Build history of the part. All positions in model axes, mm. A direction names the side the tool comes from. Round coordinates to 2 decimals unless told otherwise and drop trailing zeros. Order: outer loops, then holes, each group sorted by start corner. A loop starts at its lowest first (then second) coordinate and runs counter-clockwise, first axis right, second up. Notation, with made-up numbers: (27.5, 6) -> (78.5, 6) arc R24 ccw to (78.5, 25) -> close; hole circle Ø10 at (76.5, 80). An arc over 180 degrees is marked (long way). Answer as a JSON object with one key per item and string values.
from build123d import *

# Parameters (mm, degrees)
F1_DEPTH = 12.7
F3_D     = 12.7


# Not quite as in the source:
# - a length typed as a fraction of an inch, garbled in the dataset ("3 / 203.2 mm" for 3/8 in), is restored


with BuildPart() as f1:
    # F0 (on Front) → F1 (new body, symmetric)
    with BuildSketch(Plane.XZ):
        Polygon((0, -12.7), (0, 0), (-63.5, 0), (-63.5, 12.7), (-88.9, 12.7), (-88.9, -12.7), align=None)
    extrude(amount=F1_DEPTH, both=True)

    # F3 (through all)
    with Locations(Plane(origin=(0, 0, -12.7), x_dir=(1, 0, 0), z_dir=(0, 0, -1))):
        with Locations((-76.2, 0), (-12.7, 0)):
            Hole(F3_D / 2)


solid = f1.part
1) Probe L1, parallel to X at y = -4.5, z = -2; L2, parallel to Y at x = -76, z = 8.5; L3, parallel to X at y = 8, z = 3.75. List the from-to ranges inside material, lowest first. Write a range as from..to.
Checked values:
{"L1": "x = -88.9..-80.68, -71.72..-17.18, -8.22..0", "L2": "y = -12.7..-6.35, 6.35..12.7", "L3": "x = -88.9..-63.5"}
2) Pull direction Y, two halves, no side cores. Call faces 1 (the face through (-70, -3, 12.7)), 2 (the face through (-6.356, -0.279, -6.261)), 3 (the face through (-55, -12.7, -3)), 4 (the face through (-55, 12.7, -3)): pulls with the +Y half, pulls with the -Y half, needs draft (parallel to the pull), parting line crosses it, or undercut.
Checked values:
{"face 1": "needs draft", "face 2": "undercut", "face 3": "pulls with the -Y half", "face 4": "pulls with the +Y half"}
3) Cut at B-B, the plane y = 0. Give the cut face in (x, z), plus the area to 3 significant figures.
Checked values:
{"outline": "(-88.9, -12.7) -> (-82.55, -12.7) -> (-82.55, 12.7) -> (-88.9, 12.7) -> close; (-69.85, -12.7) -> (-19.05, -12.7) -> (-19.05, 0) -> (-63.5, 0) -> (-63.5, 12.7) -> (-69.85, 12.7) -> close; (-6.35, -12.7) -> (0, -12.7) -> (0, 0) -> (-6.35, 0) -> close", "area": "968 mm²"}
4) Cut at C-C, the plane z = 2. Give the cut face in (x, y).
Checked values:
{"outline": "(-88.9, -12.7) -> (-63.5, -12.7) -> (-63.5, 12.7) -> (-88.9, 12.7) -> close; hole circle Ø12.7 at (-76.2, 0)"}
5) Cut at A-A, the plane x = -12.7. Give the cut face in (y, z), plus the area to 3 significant figures.
Checked values:
{"outline": "(-12.7, -12.7) -> (-6.35, -12.7) -> (-6.35, 0) -> (-12.7, 0) -> close; (6.35, -12.7) -> (12.7, -12.7) -> (12.7, 0) -> (6.35, 0) -> close", "area": "161 mm²"}
6) Cut at D-D, the plane x = -76.2. Give the cut face in (y, z), plus the area to 3 significant figures.
Checked values:
{"outline": "(-12.7, -12.7) -> (-6.35, -12.7) -> (-6.35, 12.7) -> (-12.7, 12.7) -> close; (6.35, -12.7) -> (12.7, -12.7) -> (12.7, 12.7) -> (6.35, 12.7) -> close", "area": "323 mm²"}
7) Flat gauge pins, fed straight in: pin 1 Ø12 at (y, z) = (-0.5, 7) entering from +X; pin 2 Ø12 at (x, z) = (-34.5, 9) entering from +Y; pin 3 Ø12.5 at (x, y) = (-45, 4) entering from +Z. Where does each tip first touch, or does it go through?
Checked values:
{"pin 1": "stops at x = -63.5", "pin 2": "passes through", "pin 3": "stops at z = 0"}
8) Which spindle directions (+Z, -Z, +X, -X, +Y, -Y) get a long thin tool onto all of the face, cutting with end or side? Do faces 5 (the face through (-69.856, -0.279, 0.178)), 6 (the face through (-63.5, 0, 6)). Say none if no direction does.
Checked values:
{"face 5": "+Z, -Z", "face 6": "+Z, +X, +Y, -Y"}
